Input: dimensioned drawing with shaded views. Units: mm. Origin: part minimum x, y, z. A direction names the side the tool comes from. Give positions to 0.01 mm unless a question says otherwise; leave off trailing zeros. Loops run counter-clockwise (first coordinate to the right, second up) from the corner with the lowest first, then second, coordinate; pieces in that order, holes last. Notation, with made-up numbers: (22.25, 29) -> (40.25, 29) arc R35 ccw to (40.25, 67) -> close; hole circle Ø7 at (26, 73). An arc over 180 degrees is marked (long way). One line per question, with ' | ' between items. Start each with the question number.
Item 1: Set-up query: the marked faces 1, 2 and 3. Return all of +Z, -Z, +X, -X, +Y, -Y with unobstructed straight access to the full face (end or side cutting, diameter ignored); none if empty.
Item 2: Pin query (flat end, axial travel): P1, Ø4, axis at y = 31, z = 76, coming from the -X side; P2, Ø3, axis at y = 139, z = 21.5, coming from the +X side; P3, Ø1.5, axis at x = 496.5, y = 71.5, coming from the -Z side; P4, Ø2, axis at y = 161, z = 46.5, coming from the -X side. Return the tip coordinate at first contact, or that it passes through.
Item 3: Section C-C on z = 16. Return loops of the section in (x, y).
Item 4: Section A-A on y = 214.5. Return loops of the section in (x, z), then the cut area to 3 significant figures.
Item 5: Material intervals for line 1 along Z through (x, y) = (437.5, 62.5); line 2 along X through (y, z) = (163, 36.5); line 3 along X through (y, z) = (114, 101), sorted ascending. Write a range as [from, to].
Item 6: Section B-B on x = 531. Return loops of the section in (y, z), then the cut area to 3 significant figures.
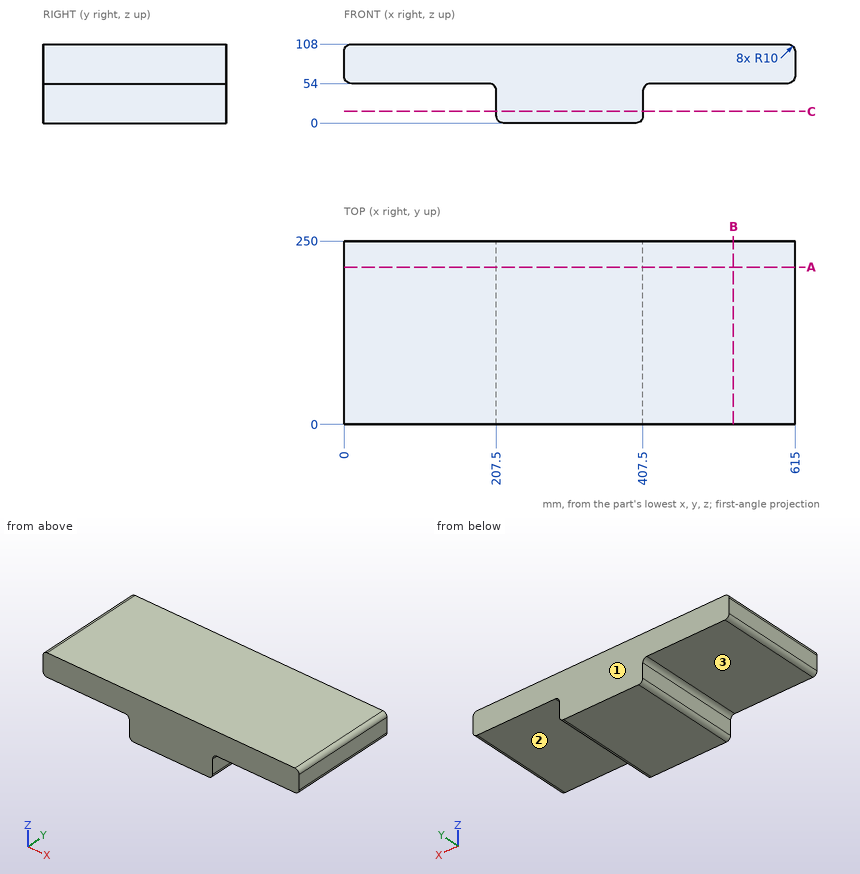
Result sheet:
1) face 1: +Z, -Z, +X, -X, +Y | face 2: -Z, +X, +Y, -Y | face 3: -Z, -X, +Y, -Y
2) P1: stops at x = 0 | P2: stops at x = 407.5 | P3: stops at z = 54 | P4: stops at x = 206.87
3) outline: (207.5, 0) -> (407.5, 0) -> (407.5, 250) -> (207.5, 250) -> close
4) outline: (0, 64) arc R10 ccw to (10, 54) -> (197.5, 54) arc R10 cw to (207.5, 44) -> (207.5, 10) arc R10 ccw to (217.5, 0) -> (397.5, 0) arc R10 ccw to (407.5, 10) -> (407.5, 44) arc R10 cw to (417.5, 54) -> (605, 54) arc R10 ccw to (615, 64) -> (615, 98) arc R10 ccw to (605, 108) -> (10, 108) arc R10 ccw to (0, 98) -> close | area: 43,900 mm²
5) line 1: z = [54, 108] | line 2: x = [207.5, 407.5] | line 3: x = [0.46, 614.54]
6) outline: (0, 54) -> (250, 54) -> (250, 108) -> (0, 108) -> close | area: 13,500 mm²
